Can you work these out from the model? Positions are in its coordinate system, mm. A direction names the side the tool comes from. Round coordinates to 2 decimals unless told otherwise and drop trailing zeros. Write each loop counter-clockwise with the first axis right and the second up, starting at its lowest first coordinate (ties: lowest second). Pieces come first, ordered by that corner, then holes. Notation, with made-up numbers: (36, 86.5) -> (75, 86.5) arc R12 cw to (75, 96.5) -> close; hole circle Ø11 at (33.5, -29). An arc over 180 degrees is marked (long way). Write item = value, one per line. Start each with the question number.
1) Imagine slicing it at D-D, the plane x = 5.75. Please give me the cut outline in (y, z).
2) I'm going to push flat-ended pins straight in: pin 1 (2.5 mm diameter, centred on y = 3.5, z = -1, fed in from -X); pin 2 (1 mm diameter, centred on x = 6, y = 2.5, fed in from +Z); pin 3 (0.6 mm diameter, centred on x = 7.5, z = 1, fed in from -Y). Where does each tip first touch, or does it pass through?
3) Thinking about a two-plate mould opening in Z: for faces 1 (the face through (-5.4, 0.9, 4.1)), 2 (the face through (0, 1, -5.8)), 3 (the face through (-2, 1.8, 0)), which applies, +Z half, -Z half, draft (parallel to the pull), parting line (faces both ways), or undercut?
4) Imagine slicing it at A-A, the plane y = 0.35. Please give me the cut outline in (x, z) (3 decimals), then the cut area to 3 significant figures.
5) For faces 4 (the face through (0.2, 3, 0)), 5 (the face through (7.294, 2.085, -4.199)), 6 (the face through (7.294, 2.101, 4.215)), which set-ups out of +Z, -Z, +X, -X, +Y, -Y let a thin tool reach every point of the face, with its end or its side?
6) Imagine slicing it at B-B, the plane x = -5.9. Please give me the cut outline in (y, z) (3 decimals), then the cut area to 3 significant figures.
7) If I drill on line 1 (Y direction, x = -0.5, z = 1.25); line 2 (X direction, y = 3.25, z = -2.5); line 3 (X direction, y = 1.75, z = 1.25), over which ranges is the centre line in solid material (lowest first)?
8) Imagine slicing it at C-C, the plane z = 4.25. Please give me the cut outline in (x, y).
from build123d import *

# Parameters (mm, degrees)
SKETCH_1_W          = 13.8
SKETCH_1_H          = 11.6
EXTRUDE_1_DEPTH     = 1.8
EXTRUDE_START       = -1.8
SKETCH_4_W          = 7.5
SKETCH_4_H          = 9
EXTRUDE_2_DEPTH     = 4.9
SKETCH_5_W          = 9
SKETCH_5_H          = 1.8
CUT_EXTRUDE_1_DEPTH = 0.8
FILLET_1_R          = 1
CUT_EXTRUDE_2_REACH = 12.126
SKETCH_6_R          = 0.5


with BuildPart() as part:
    # 草图1 → 凸台-拉伸1 (new body)
    with BuildSketch(Plane(origin=(0, 0, 0), x_dir=(1, 0, 0), z_dir=(0, 1, 0))):
        Rectangle(SKETCH_1_W, SKETCH_1_H)
    extrude(amount=EXTRUDE_1_DEPTH)

    # 草图4 → 凸台-拉伸2 (add)
    with BuildSketch(Plane(origin=(0, 1.8, 0), x_dir=(1, 0, 0), z_dir=(0, 1, 0)).offset(EXTRUDE_START)):
        with Locations((3.95, 0)):
            Rectangle(SKETCH_4_W, SKETCH_4_H)
    extrude(amount=EXTRUDE_2_DEPTH)

    # 草图5 → 切除-拉伸1 (cut)
    with BuildSketch(Plane(origin=(7.7, 0, 0), x_dir=(0, 0, -1), z_dir=(1, 0, 0))):
        with Locations((0, 0.9)):
            Rectangle(SKETCH_5_W, SKETCH_5_H)
    extrude(amount=-CUT_EXTRUDE_1_DEPTH, mode=Mode.SUBTRACT)

    # 圆角1
    fillet_1_edges = [part.edges().sort_by_distance(p)[0] for p in [
        (3.95, 4.9, 4.5),
        (3.95, 4.9, -4.5),
        (7.3, 1.8, -4.5),
        (7.3, 1.8, 4.5),
    ]]
    fillet(fillet_1_edges, radius=FILLET_1_R)

    # 草图6 → 切除-拉伸2 (cut, up to next)
    with BuildSketch(Plane(origin=(0, 1.8, 0), x_dir=(1, 0, 0), z_dir=(0, 1, 0)), mode=Mode.PRIVATE) as cut_extrude_2_sk1:
        with Locations(Location((-5.9, 4.125, 0), (0, 0, 270))):
            Circle(SKETCH_6_R)
    cut_extrude_2_tool1 = extrude(cut_extrude_2_sk1.sketch, amount=-CUT_EXTRUDE_2_REACH, mode=Mode.PRIVATE) & part.part
    # 草图6 → 切除-拉伸2 (cut, up to next)
    with BuildSketch(Plane(origin=(0, 1.8, 0), x_dir=(1, 0, 0), z_dir=(0, 1, 0)), mode=Mode.PRIVATE) as cut_extrude_2_sk2:
        with Locations(Location((-5.9, 1.375, 0), (0, 0, 270))):
            Circle(SKETCH_6_R)
    cut_extrude_2_tool2 = extrude(cut_extrude_2_sk2.sketch, amount=-CUT_EXTRUDE_2_REACH, mode=Mode.PRIVATE) & part.part
    # 草图6 → 切除-拉伸2 (cut, up to next)
    with BuildSketch(Plane(origin=(0, 1.8, 0), x_dir=(1, 0, 0), z_dir=(0, 1, 0)), mode=Mode.PRIVATE) as cut_extrude_2_sk3:
        with Locations(Location((-5.9, -1.375, 0), (0, 0, 270))):
            Circle(SKETCH_6_R)
    cut_extrude_2_tool3 = extrude(cut_extrude_2_sk3.sketch, amount=-CUT_EXTRUDE_2_REACH, mode=Mode.PRIVATE) & part.part
    # 草图6 → 切除-拉伸2 (cut, up to next)
    with BuildSketch(Plane(origin=(0, 1.8, 0), x_dir=(1, 0, 0), z_dir=(0, 1, 0)), mode=Mode.PRIVATE) as cut_extrude_2_sk4:
        with Locations(Location((-5.9, -4.125, 0), (0, 0, 270))):
            Circle(SKETCH_6_R)
    cut_extrude_2_tool4 = extrude(cut_extrude_2_sk4.sketch, amount=-CUT_EXTRUDE_2_REACH, mode=Mode.PRIVATE) & part.part
    add(cut_extrude_2_tool1.solids().sort_by_distance((-5.9, 1.8, -4.125))[0], mode=Mode.SUBTRACT)
    add(cut_extrude_2_tool2.solids().sort_by_distance((-5.9, 1.8, -1.375))[0], mode=Mode.SUBTRACT)
    add(cut_extrude_2_tool3.solids().sort_by_distance((-5.9, 1.8, 1.375))[0], mode=Mode.SUBTRACT)
    add(cut_extrude_2_tool4.solids().sort_by_distance((-5.9, 1.8, 4.125))[0], mode=Mode.SUBTRACT)


solid = part.part
Reported:
q1.outline = (0, -5.8) -> (1.8, -5.8) -> (1.8, -4.5) -> (3.9, -4.5) arc R1 ccw to (4.9, -3.5) -> (4.9, 3.5) arc R1 ccw to (3.9, 4.5) -> (1.8, 4.5) -> (1.8, 5.8) -> (0, 5.8) -> close
q2.pin_1 = 0.2
q2.pin_2 = 4.5
q2.pin_3 = 1.8
q3.face_1 = undercut
q3.face_2 = -Z half
q3.face_3 = draft
q4.outline = (-6.9, -5.8) -> (6.9, -5.8) -> (6.9, 5.8) -> (-6.9, 5.8) -> close; hole circle Ø1 at (-5.9, -4.125); hole circle Ø1 at (-5.9, -1.375); hole circle Ø1 at (-5.9, 1.375); hole circle Ø1 at (-5.9, 4.125)
q4.area = 157 mm²
q5.face_4 = +Z, -Z, -X, +Y
q5.face_5 = -Z, +X, -Y
q5.face_6 = +Z, +X, -Y
q6.outline = (0, -5.8) -> (1.8, -5.8) -> (1.8, -4.625) -> (0, -4.625) -> close; (0, -3.625) -> (1.8, -3.625) -> (1.8, -1.875) -> (0, -1.875) -> close; (0, -0.875) -> (1.8, -0.875) -> (1.8, 0.875) -> (0, 0.875) -> close; (0, 1.875) -> (1.8, 1.875) -> (1.8, 3.625) -> (0, 3.625) -> close; (0, 4.625) -> (1.8, 4.625) -> (1.8, 5.8) -> (0, 5.8) -> close
q6.area = 13.7 mm²
q7.line_1 = 0 to 1.8
q7.line_2 = 0.2 to 7.7
q7.line_3 = -6.9 to -6.38, -5.42 to 6.9
q8.outline = (-6.9, 0) -> (-6.38, 0) -> (-6.38, 1.8) -> (-6.9, 1.8) -> close; (-5.42, 0) -> (6.9, 0) -> (6.9, 2.14) -> (7.7, 2.14) -> (7.7, 4.56) -> (0.2, 4.56) -> (0.2, 1.8) -> (-5.42, 1.8) -> close
